The drawing under review shows one solid part. Ordinate dimensions are in mm from its lowest x, y, z. Coordinates: 2 decimals unless noted, no trailing zeros. Order: outer loops, then holes, each group sorted by start corner. A loop starts at its lowest first (then second) coordinate and runs counter-clockwise, first axis right, second up. Notation, with made-up numbers: (10, 84.25) -> (67, 84.25) arc R23 ccw to (67, 119.25) -> close; hole circle Ø11 at (36.25, 79.5). An arc over 180 degrees is marked (long way). Use a Markdown table: item, result. Add a question column.
Q1. Wall thickness on probe 1 along Y at (x, z) = (2.75, 8) (1 decimal); probe 2 along Y at (x, z) = (8.5, 8) (1 decimal); probe 3 along X at (y, z) = (4, 1): over which ranges is each line inside the solid? List them lowest first.
Q2. The part is to be moulded in two halves that separate along X. For the marked faces 1, 2, 3 and 4, say which applies: pulls with the +X half, pulls with the -X half, needs draft (parallel to the pull), parting line crosses it, or undercut.
Q3. Add section D-D (z = 6.5). State the section outline as (x, y) points (1 decimal), then the cut area to 3 significant figures.
Q4. Insertion check: pin 1 (1 mm diameter, centred on y = 7.5, z = 4, fed in from +X); pin 2 (3 mm diameter, centred on x = 8.5, z = 9, fed in from -Y); pin 3 (1.5 mm diameter, centred on x = 8, z = 5, fed in from +Y) (1 decimal). Each pin has a flat end and moves straight along its axis. Give the tip position at first contact, or say it passes through.
Q5. Add section C-C (x = 6.75). State the section outline as (y, z) points.
Q6. Add section B-B (y = 6.75). State the section outline as (x, z) points.
Q7. Add section A-A (z = 1). State the section outline as (x, y) points.
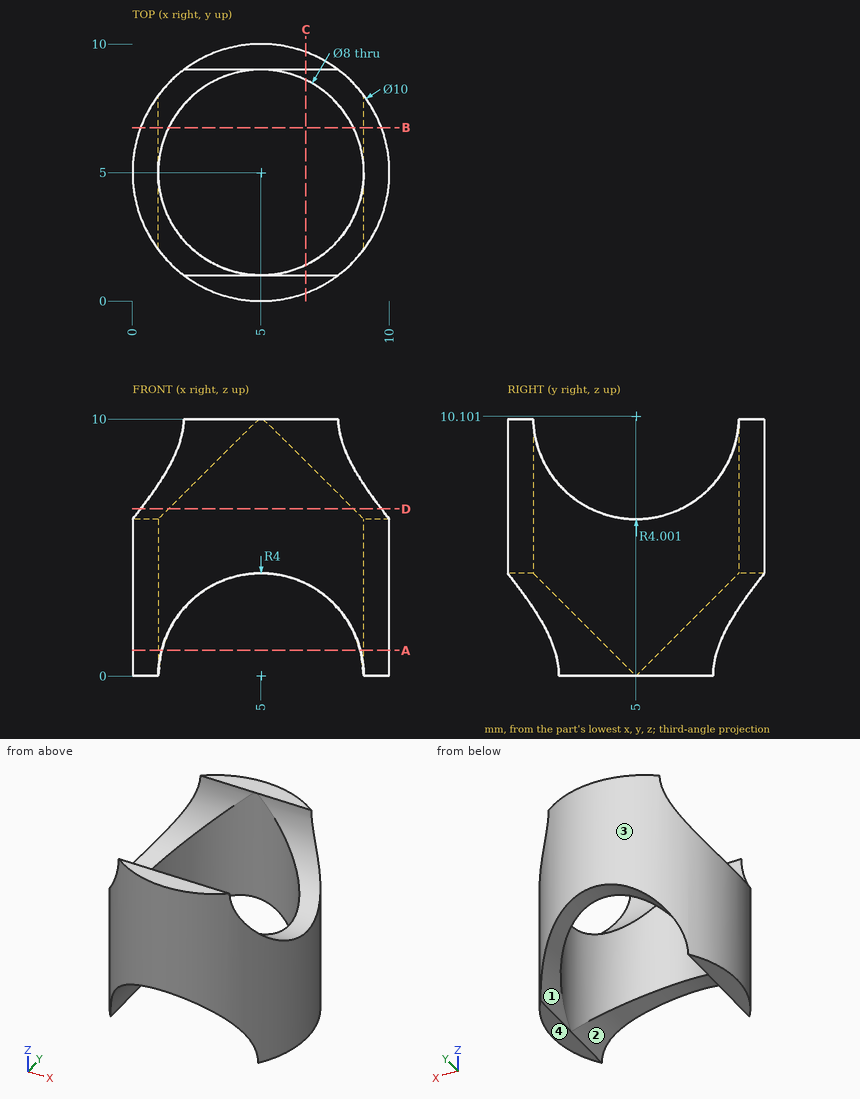
Established:
| question | item | result |
|---|---|---|
| 1 | probe 1 | 0.5 to 1.6, 8.4 to 9.5 |
| 1 | probe 2 | 1.4 to 1.6, 8.4 to 8.6 |
| 1 | probe 3 | 0.1 to 1.13, 8.87 to 9.9 |
| 2 | face 1 | undercut |
| 2 | face 2 | undercut |
| 2 | face 3 | parting line crosses it |
| 2 | face 4 | needs draft |
| 3 | outline | (0.3, 3.3) arc R5 ccw to (9.7, 3.3) -> (8.6, 3.3) arc R4 cw to (1.4, 3.3) -> close; (0.3, 6.7) -> (1.4, 6.7) arc R4 cw to (8.6, 6.7) -> (9.7, 6.7) arc R5 ccw to start |
| 3 | area | 21.1 mm^2 |
| 4 | pin 1 | x = 9.58 |
| 4 | pin 2 | y = 0.42 |
| 4 | pin 3 | y = 9.5 |
| 5 | outline | (0.32, 3.6) -> (1.4, 3.6) -> (1.4, 8.35) arc R4 cw to (1, 10) -> (0.32, 10) -> close; (8.6, 3.6) -> (9.68, 3.6) -> (9.68, 10) -> (9, 10) arc R4 cw to (8.6, 8.35) -> close |
| 6 | outline | (0.32, 0) -> (1, 0) arc R4 cw to (1.4, 1.75) -> (1.4, 6.5) -> (0.32, 6.5) -> close; (8.6, 1.75) arc R4 cw to (9, 0) -> (9.68, 0) -> (9.68, 6.5) -> (8.6, 6.5) -> close |
| 7 | outline | (1.13, 1.84) -> (1.13, 4) arc R4 cw to (1.13, 6) -> (1.13, 8.16) arc R5 ccw to start; (8.87, 1.84) arc R5 ccw to (8.87, 8.16) -> (8.87, 6) arc R4 cw to (8.87, 4) -> close |
